Input: part model. Units: mm. Frame: model coordinates. Face numbers are marked on the shaded views. A direction names the side the tool comes from. Coordinates: 2 decimals unless noted, no trailing zeros. Write each loop counter-clockwise with the first axis right and the second up, starting at its lowest first coordinate (ties: lowest second). Pieces come first, ordered by that corner, then holes. Notation, with made-up numbers: (65, 32.5) -> (114, 32.5) arc R23 ccw to (114, 48.5) -> close; hole circle Ø10 at (63.25, 4). An arc over 180 degrees is marked (long way). Use one line per item in the form item = value. Start each with the question number.
(1) Cut plane B-B on y = 0. Return the cut outline in (x, z), plus the area to 3 significant figures.
(2) First-contact query: pin 1 (4 mm diameter, centred on y = -6, z = -3, fed in from -X); pin 2 (1.3 mm diameter, centred on x = -10, z = -1, fed in from +Y); pin 3 (1.5 mm diameter, centred on x = 0, z = -6, fed in from -Y); pin 4 (4 mm diameter, centred on x = 9.906, y = 0, fed in from -Z). Flat tips, straight axial feed; report the tip coordinate or a pass-through.
(3) Ray query, line 1 along Y through (x, z) = (9.25, -0.25); line 2 along Y through (x, z) = (7, -5); line 3 along Y through (x, z) = (10.25, -0.25). Return the intervals inside material, ascending.
(4) Cut plane C-C on z = -0.75. Return the cut outline in (x, y).
(5) Cut plane A-A on x = -3. Return the cut outline in (y, z), plus the area to 3 significant figures.
(6) Set-up query: the marked faces 1 and 2. Return all of +Z, -Z, +X, -X, +Y, -Y with unobstructed straight access to the full face (end or side cutting, diameter ignored); none if empty.
(7) Cut plane D-D on y = 4.75. Return the cut outline in (x, z), plus the area to 3 significant figures.
```python
from build123d import *

# Parameters (mm, degrees)
SKETCH2_W              = 27.94
SKETCH2_H              = 20.2692
BOSS_EXTRUDE2_DEPTH    = 8.128
DRAFT1_ANGLE           = 0.5
CONVERT_SOLID1_START   = -13.97
CONVERT_SOLID1_DEPTH   = 27.94
CONVERT_SOLID1_2_DEPTH = 27.94
SKETCH26_R             = 0.6604
CUT_EXTRUDE6_DEPTH     = 27.664739949
SKETCH16_R             = 1.2192
SKETCH16_W             = 4.064
SKETCH16_H             = 2.794
CUT_EXTRUDE4_DEPTH     = 60.515150005
SKETCH35_W             = 11.684
SKETCH35_H             = 9.271
CUT_EXTRUDE7_DEPTH     = 3.81
CHAMFER1_SIZE          = 2.286


# Read off the part's stored shape, not the designer's step: Convert-Solid1
with BuildPart() as part:
    # Sketch2 → Boss-Extrude2 (new body)
    with BuildSketch(Plane.XY):
        with Locations((0, -1.8034)):
            Rectangle(SKETCH2_W, SKETCH2_H)
    extrude(amount=-BOSS_EXTRUDE2_DEPTH)

    # Draft1
    draft1_faces = [part.faces().sort_by_distance(p)[0] for p in [
        (0, 8.3312, -4.064),
    ]]
    draft(draft1_faces, Plane.XY.offset(-5.08), DRAFT1_ANGLE)

    # Convert-Solid1 outline → Convert-Solid1 (cut)
    with BuildSketch(Plane.YZ.offset(CONVERT_SOLID1_START)):
        with BuildLine():
            Line((-11.938, -8.128), (7.138553067, -8.128))
            Line((7.138553067, -8.128), (7.084852727, -1.97455038))
            ThreePointArc((7.084852727, -1.97455038), (6.859340961, -1.440038744), (6.322881741, -1.2192))
            Line((6.322881741, -1.2192), (-11.938, -1.2192))
            Line((-11.938, -1.2192), (-11.938, -8.128))
        make_face()
        with BuildLine():
            ThreePointArc((6.322881741, 0), (7.717675713, -0.574180734), (8.304006303, -1.963910988))
            Line((8.304006303, -1.963910988), (8.286867512, 0))
            Line((8.286867512, 0), (6.322881741, 0))
        make_face()
    extrude(amount=CONVERT_SOLID1_DEPTH, mode=Mode.SUBTRACT)

    # Convert-Solid1 2 outline → Convert-Solid1 2 (add)
    with BuildSketch(Plane.YZ.offset(CONVERT_SOLID1_START)):
        Polygon((7.138553067, -8.128), (7.138645916, -8.138639392), (8.357799493, -8.128), align=None)
    extrude(amount=CONVERT_SOLID1_2_DEPTH)

    # Sketch26 → Cut-Extrude6 (cut, through all)
    with BuildSketch(Plane(origin=(0, 8.375524998, -10.159141632), x_dir=(1, 0, 0), z_dir=(0, -0.9999619230641713, -0.008726535498373954))):
        with Locations(Location((9.652, 5.079528476, 0), (0, 0, 270))):
            Circle(SKETCH26_R)
        Polygon((9.887639275, 0.235167751), (15.766051224, 6.1135797), (15.766051224, 0.235167751), align=None)
    cut_extrude6 = extrude(amount=CUT_EXTRUDE6_DEPTH, mode=Mode.SUBTRACT)

    # Sketch16 → Cut-Extrude4 (cut, through all)
    with BuildSketch(Plane(origin=(0, 45.339, 0), x_dir=(1, 0, 0), z_dir=(0, 0, -1))):
        with Locations(Location((9.906, 45.339, 0), (0, 0, 180))):
            Circle(SKETCH16_R)
        with Locations((10.16, 50.8)):
            Rectangle(SKETCH16_W, SKETCH16_H)
    cut_extrude4 = extrude(amount=CUT_EXTRUDE4_DEPTH, mode=Mode.SUBTRACT)

    # Mirror1: Cut-Extrude6, Cut-Extrude4 across plane
    add(cut_extrude6.mirror(Plane(origin=(0, 0, 0), x_dir=(0, 0, 1), z_dir=(1, 0, 0))), mode=Mode.SUBTRACT)
    add(cut_extrude4.mirror(Plane(origin=(0, 0, 0), x_dir=(0, 0, 1), z_dir=(1, 0, 0))), mode=Mode.SUBTRACT)

    # Sketch35 → Cut-Extrude7 (cut)
    with BuildSketch(Plane.XY):
        with Locations((0, -2.2225)):
            Rectangle(SKETCH35_W, SKETCH35_H)
    extrude(amount=-CUT_EXTRUDE7_DEPTH, mode=Mode.SUBTRACT)

    # Chamfer1
    chamfer1_edges = [part.edges().sort_by_distance(p)[0] for p in [
        (13.97, -11.938, -0.6096),
        (-13.97, -11.938, -0.6096),
    ]]
    chamfer(chamfer1_edges, length=CHAMFER1_SIZE)


solid = part.part
```
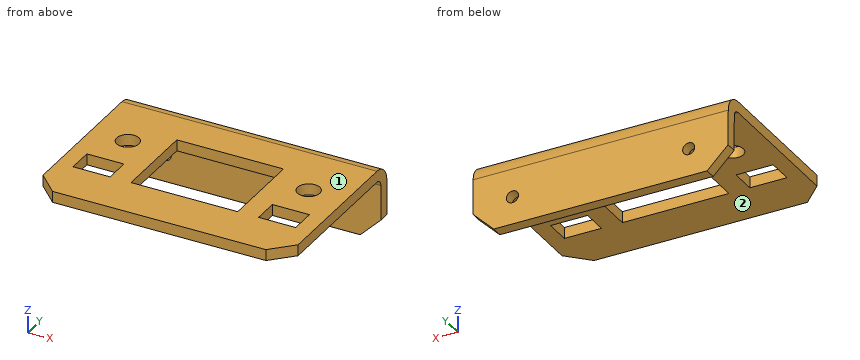
Values:
q1.outline = (-13.97, -1.22) -> (-11.13, -1.22) -> (-11.13, 0) -> (-13.97, 0) -> close; (-8.69, -1.22) -> (-5.84, -1.22) -> (-5.84, 0) -> (-8.69, 0) -> close; (5.84, -1.22) -> (8.69, -1.22) -> (8.69, 0) -> (5.84, 0) -> close; (11.13, -1.22) -> (13.97, -1.22) -> (13.97, 0) -> (11.13, 0) -> close
q1.area = 13.9 mm2
q2.pin_1 = -13.97
q2.pin_2 = 8.28
q2.pin_3 = 7.11
q2.pin_4 = -1.22
q3.line_1 = -11.94 to -6.86, -4.06 to -1.03, 1.03 to 7.29
q3.line_2 = 7.11 to 8.33
q3.line_3 = -11.94 to -6.86, -4.06 to -1.17, 1.17 to 7.29
q4.outline = (-13.97, -9.65) -> (-11.68, -11.94) -> (11.68, -11.94) -> (13.97, -9.65) -> (13.97, 7.88) -> (-13.97, 7.88) -> close; hole (-12.19, -6.86) -> (-8.13, -6.86) -> (-8.13, -4.06) -> (-12.19, -4.06) -> close; hole circle Ø2.44 at (-9.91, 0); hole (-5.84, -6.86) -> (5.84, -6.86) -> (5.84, 2.41) -> (-5.84, 2.41) -> close; hole (8.13, -6.86) -> (12.19, -6.86) -> (12.19, -4.06) -> (8.13, -4.06) -> close; hole circle Ø2.44 at (9.91, 0)
q5.outline = (-11.94, -1.22) -> (-6.86, -1.22) -> (-6.86, 0) -> (-11.94, 0) -> close; (2.41, -1.22) -> (6.32, -1.22) arc R0.76 cw to (7.08, -1.97) -> (7.14, -8.14) -> (8.36, -8.13) -> (8.3, -1.96) arc R1.98 ccw to (6.32, 0) -> (2.41, 0) -> close
q5.area = 21.1 mm2
q6.face_1 = +Z, +X, -X, +Y, -Y
q6.face_2 = -Z, +X, -X, -Y
q7.outline = (-13.97, -1.22) -> (13.97, -1.22) -> (13.97, 0) -> (-13.97, 0) -> close
q7.area = 34.1 mm2
